Input: part model. Units: mm. Frame: model coordinates. A direction names the side the tool comes from. Round coordinates to 2 decimals unless told otherwise and drop trailing zeros. Order: outer loops, then holes, each group sorted by start corner. A loop starts at its lowest first (then second) coordinate and runs counter-clockwise, first axis right, second up.
Item 1: Mould query, pull axis X, two halves, no side actions, for faces 3 (the cylindrical face through (54.894, 5.972, 0.24)), 4 (the cylindrical face through (-9, 2, 0)), 5 (the flat face through (16, 0, 0)). Classes: released by +X, released by -X, zero draft, split by the parting line, or undercut.
Item 2: First-contact query: pin 1 (4 mm diameter, centred on x = 18, z = 0, fed in from +Y); pin 2 (1.8 mm diameter, centred on x = 0, z = 0, fed in from -Y); pin 3 (2 mm diameter, centred on y = 3, z = -2.5, fed in from -X); pin 4 (1.5 mm diameter, centred on x = 19.5, y = 3, fed in from -Z). Flat tips, straight axial feed; report the tip coordinate or a pass-through.
Item 3: Cut plane B-B on y = 6.75. Output: boundary loops of the cut face in (x, z).
Item 4: Cut plane A-A on z = 0. Output: boundary loops of the cut face in (x, y), then the cut area to 3 significant figures.
Item 5: Line query: L1, parallel to X at y = 5.85, z = 0; L2, parallel to Z at x = 49.9, y = 1.2; L3, parallel to Z at x = 49.9, y = 5.85. Output: solid intervals per line, ascending.
Item 6: Reachability of faces 1 (the flat face through (0, 8, -2)), 2 (the cylindrical face through (-0.33, 5.972, 7.493)) from +Z, -Z, +X, -X, +Y, -Y: full face, straight path, thin tool, end or side. Return the list, or none.
```python
from build123d import *

# Parameters (mm, degrees)
SKETCH_1_R      = 1.5
SKETCH_1_R_2    = 3.4
EXTRUDE_1_DEPTH = 4
FILLET_1_R      = 0.5
SKETCH_2_R      = 7.5
SKETCH_2_R_2    = 1.5
SKETCH_2_R_3    = 5
SKETCH_2_R_4    = 3.4
EXTRUDE_2_DEPTH = 4


with BuildPart() as part:
    # 草图1 → 凸台-拉伸1 (new body)
    with BuildSketch(Plane(origin=(0, 0, 0), x_dir=(1, 0, 0), z_dir=(0, 1, 0))):
        with BuildLine():
            ThreePointArc((2.718196527, 8.579709065), (-9, 0), (2.718196527, -8.579709065))
            ThreePointArc((2.718196527, -8.579709065), (25.653399298, -4.228021884), (48.967323861, -5.420342722))
            ThreePointArc((48.967323861, -5.420342722), (55.4, 0), (48.967323861, 5.420342722))
            ThreePointArc((48.967323861, 5.420342722), (25.653399298, 4.228021884), (2.718196527, 8.579709065))
        make_face()
        with Locations(Location((0, 0, 0), (0, 0, 270))):
            Circle(SKETCH_1_R, mode=Mode.SUBTRACT)
        with Locations(Location((49.9, 0, 0), (0, 0, 270))):
            Circle(SKETCH_1_R_2, mode=Mode.SUBTRACT)
    extrude(amount=EXTRUDE_1_DEPTH)

    # 圆角1
    fillet_1_edges = [part.edges().sort_by_distance(p)[0] for p in [
        (25.653399298, 4, 4.228021884),
        (55.4, 4, 0),
        (25.653399298, 4, -4.228021884),
        (55.4, 0, 0),
        (25.653399298, 0, 4.228021884),
        (-9, 0, 0),
        (25.653399298, 0, -4.228021884),
        (-9, 4, 0),
    ]]
    fillet(fillet_1_edges, radius=FILLET_1_R)

    # 草图2 → 凸台-拉伸2 (add)
    # profile 1 of 2: a face of its own
    with BuildSketch(Plane(origin=(0, 4, 0), x_dir=(1, 0, 0), z_dir=(0, 1, 0))):
        with Locations(Location((0, 0, 0), (0, 0, 90))):
            Circle(SKETCH_2_R)
        with Locations(Location((0, 0, 0), (0, 0, 90))):
            Circle(SKETCH_2_R_2, mode=Mode.SUBTRACT)
    # profile 2 of 2: a face of its own
    with BuildSketch(Plane(origin=(0, 4, 0), x_dir=(1, 0, 0), z_dir=(0, 1, 0))):
        with Locations(Location((49.9, 0, 0), (0, 0, 99.763253754))):
            Circle(SKETCH_2_R_3)
        with Locations(Location((49.9, 0, 0), (0, 0, 90))):
            Circle(SKETCH_2_R_4, mode=Mode.SUBTRACT)
    extrude(amount=EXTRUDE_2_DEPTH)


solid = part.part
```
From the geometry:
1. face 3: undercut
1. face 4: split by the parting line
1. face 5: zero draft
2. pin 1: stops at y = 4
2. pin 2: passes through
2. pin 3: stops at x = -8.87
2. pin 4: stops at z = -4.95
3. outline: circle Ø15 at (0, 0); circle Ø10 at (49.9, 0); hole circle Ø3 at (0, 0); hole circle Ø6.8 at (49.9, 0)
4. outline: (-9, 0.5) arc R0.5 ccw to (-8.5, 0) - (-1.5, 0) - (-1.5, 8) - (-7.5, 8) - (-7.5, 4) - (-8.5, 4) arc R0.5 ccw to (-9, 3.5) - close; (1.5, 0) - (46.5, 0) - (46.5, 8) - (44.9, 8) - (44.9, 4) - (7.5, 4) - (7.5, 8) - (1.5, 8) - close; (53.3, 0) - (54.9, 0) arc R0.5 ccw to (55.4, 0.5) - (55.4, 3.5) arc R0.5 ccw to (54.9, 4) - (54.9, 8) - (53.3, 8) - close
4. area: 279 mm2
5. L1: x = -7.5 to -1.5, 1.5 to 7.5, 44.9 to 46.5, 53.3 to 54.9
5. L2: z = -5.5 to -3.4, 3.4 to 5.5
5. L3: z = -5 to -3.4, 3.4 to 5
6. face 1: +Z, -Z, +X, -X, +Y
6. face 2: +Y
